Verification items for the finished model (mm, model axes). Round coordinates to 2 decimals unless told otherwise and drop trailing zeros. Order: outer loops, then holes, each group sorted by start corner. A loop starts at its lowest first (then second) coordinate and runs counter-clockwise, first axis right, second up. Notation, with made-up numbers: (-28.5, 9) -> (-8.5, 9) arc R6 ccw to (-8.5, 15) -> close; hole circle Ø3 at (89, 79). An arc over 180 degrees is marked (long way). Write item = value, one per line. Start each with the question number.
from build123d import *

# Parameters (mm, degrees)
F0_R     = 1.37362
F0_R_2   = 0.635
F0_R_3   = 0.4064
F0_R_4   = 0.508
F1_DEPTH = 25.4


with BuildPart() as f1:
    # F0 (on Front) → F1 (new body)
    with BuildSketch(Plane.XZ):
        Circle(F0_R)
        with Locations((0, -0.63702)):
            Circle(F0_R_2, mode=Mode.SUBTRACT)
        with Locations((-0.857486, 0.11839)):
            Circle(F0_R_3, mode=Mode.SUBTRACT)
        with Locations((0, 0.60758)):
            Circle(F0_R_4, mode=Mode.SUBTRACT)
        with Locations((0.857486, 0.11839)):
            Circle(F0_R_3, mode=Mode.SUBTRACT)
    extrude(amount=F1_DEPTH)


solid = f1.part
(1) Cross-section at B-B (y = -9.5). Enter the section's corners in (x, z) (3 decimals), and give its area (3 significant figures).
(2) Scan lines: line 1 along X through (y, z) = (-6.75, -0.1); line 2 along Z through (x, y) = (0.55, -12.75); line 3 along X through (y, z) = (-19.25, -0.5). Record each from-to range of solid material in increasing order. Write a range as from..to.
(3) Draft check along X on faces 1 (the cylindrical face through (0.8, -12.52, 0.52)), 2 (the cylindrical face through (-0.18, -12.52, 1.36)), 3 (the cylindrical face through (-1.157, -12.522, 0.393)). Enter one of: +X half, -X half, draft (parallel to the pull), parting line (faces both ways), or undercut.
(4) Depth check by flat-ended pin: pin 1 (1 mm diameter, centred on y = -18.5, z = 1, fed in from -X); pin 2 (1 mm diameter, centred on x = 0, z = -0.64, fed in from +Y); pin 3 (1 mm diameter, centred on x = -1, z = 0.5, fed in from +Y). Enter the tip coordinate at first touch or a pass-through.
(5) Cross-section at A-A (x = 0). Enter the section's corners in (y, z), and give its area (3 significant figures).
Outcome:
q1.outline = circle Ø2.747 at (0, 0); hole circle Ø0.813 at (-0.857, 0.118); hole circle Ø1.27 at (0, -0.637); hole circle Ø1.016 at (0, 0.608); hole circle Ø0.813 at (0.857, 0.118)
q1.area = 2.81 mm^2
q2.line_1 = -1.37..-1.2, -0.51..-0.34, 0.34..0.51, 1.2..1.37
q2.line_2 = -1.26..-0.95, -0.32..-0.15, 0.38..1.26
q2.line_3 = -1.28..-0.62, 0.62..1.28
q3.face_1 = undercut
q3.face_2 = parting line
q3.face_3 = undercut
q4.pin_1 = -1.28
q4.pin_2 = through
q4.pin_3 = 0
q5.outline = (-25.4, -1.37) -> (0, -1.37) -> (0, -1.27) -> (-25.4, -1.27) -> close; (-25.4, 0) -> (0, 0) -> (0, 0.1) -> (-25.4, 0.1) -> close; (-25.4, 1.12) -> (0, 1.12) -> (0, 1.37) -> (-25.4, 1.37) -> close
q5.area = 11.7 mm^2
